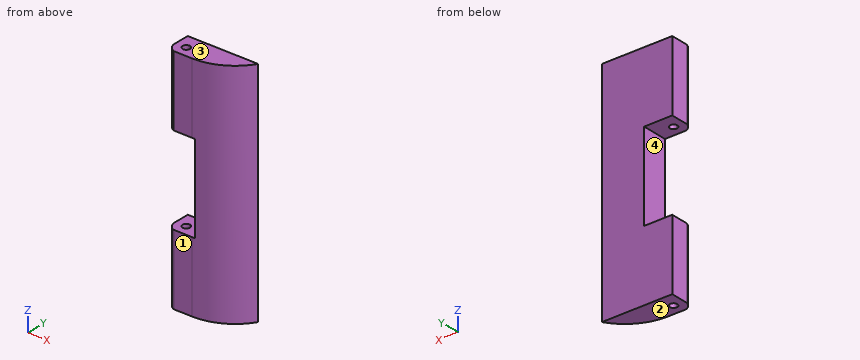
```python
from build123d import *

# Parameters (mm, degrees)
F0_W        = 24
F0_H        = 14.5
F1_DEPTH    = 130
F2_DEPTH    = 130
F3_DEPTH    = 90
F4_DEPTH    = 40
F5_R        = 1
F6_T1_DEPTH = 258.4279953904


# Not quite as in the source:
# - a fillet or chamfer that OpenCascade refuses, or shapes differently, is made with other operations: its cross-section is extruded or revolved along the edge and cut away or added


with BuildPart() as f1:
    # F0 (on Top) → F1 (new body)
    with BuildSketch(Plane.XY):
        with Locations((21.9, 1.16)):
            Rectangle(F0_W, F0_H)
    extrude(amount=F1_DEPTH)

    # F0 (on Top) → F2 (join)
    with BuildSketch(Plane.XY):
        with BuildLine():
            Line((9.9, 8.41), (6.1, 8.41))
            Line((6.1, 8.41), (6.1, -1.59))
            ThreePointArc((6.1, -1.59), (4.7073896383, -4.2954889128), (2.25, -6.09))
            Line((2.25, -6.09), (9.9, -6.09))
            Line((9.9, -6.09), (9.9, 8.41))
        make_face()
        with BuildLine():
            Line((6.1, -1.59), (6.1, 8.41))
            Line((6.1, 8.41), (0, 8.41))
            Line((0, 8.41), (0, 2.15))
            ThreePointArc((0, 2.15), (1.5202795796, 1.5202795796), (2.15, 0))
            ThreePointArc((2.15, 0), (1.5202795796, -1.5202795796), (0, -2.15))
            Line((0, -2.15), (0, -6.09))
            Line((0, -6.09), (2.25, -6.09))
            ThreePointArc((2.25, -6.09), (4.7073896383, -4.2954889128), (6.1, -1.59))
        make_face()
        with BuildLine():
            Line((0, 2.15), (0, 8.41))
            Line((0, 8.41), (-6.1, 8.41))
            Line((-6.1, 8.41), (-6.1, -1.59))
            ThreePointArc((-6.1, -1.59), (-4.7073896383, -4.2954889128), (-2.25, -6.09))
            Line((-2.25, -6.09), (0, -6.09))
            Line((0, -6.09), (0, -2.15))
            ThreePointArc((0, -2.15), (-2.15, 0), (0, 2.15))
        make_face()
    extrude(amount=F2_DEPTH)

    # F0 (on Top) → F3 (cut)
    with BuildSketch(Plane.XY):
        with BuildLine():
            Line((9.9, 8.41), (6.1, 8.41))
            Line((6.1, 8.41), (6.1, -1.59))
            ThreePointArc((6.1, -1.59), (4.7073896383, -4.2954889128), (2.25, -6.09))
            Line((2.25, -6.09), (9.9, -6.09))
            Line((9.9, -6.09), (9.9, 8.41))
        make_face()
        with BuildLine():
            Line((6.1, -1.59), (6.1, 8.41))
            Line((6.1, 8.41), (0, 8.41))
            Line((0, 8.41), (0, 2.15))
            ThreePointArc((0, 2.15), (1.5202795796, 1.5202795796), (2.15, 0))
            ThreePointArc((2.15, 0), (1.5202795796, -1.5202795796), (0, -2.15))
            Line((0, -2.15), (0, -6.09))
            Line((0, -6.09), (2.25, -6.09))
            ThreePointArc((2.25, -6.09), (4.7073896383, -4.2954889128), (6.1, -1.59))
        make_face()
        with BuildLine():
            Line((0, 2.15), (0, 8.41))
            Line((0, 8.41), (-6.1, 8.41))
            Line((-6.1, 8.41), (-6.1, -1.59))
            ThreePointArc((-6.1, -1.59), (-4.7073896383, -4.2954889128), (-2.25, -6.09))
            Line((-2.25, -6.09), (0, -6.09))
            Line((0, -6.09), (0, -2.15))
            ThreePointArc((0, -2.15), (-2.15, 0), (0, 2.15))
        make_face()
    extrude(amount=F3_DEPTH, mode=Mode.SUBTRACT)

    # F0 (on Top) → F4 (join)
    with BuildSketch(Plane.XY):
        with BuildLine():
            Line((0, 2.15), (0, 8.41))
            Line((0, 8.41), (-6.1, 8.41))
            Line((-6.1, 8.41), (-6.1, -1.59))
            ThreePointArc((-6.1, -1.59), (-4.7073896383, -4.2954889128), (-2.25, -6.09))
            Line((-2.25, -6.09), (0, -6.09))
            Line((0, -6.09), (0, -2.15))
            ThreePointArc((0, -2.15), (-2.15, 0), (0, 2.15))
        make_face()
        with BuildLine():
            Line((6.1, -1.59), (6.1, 8.41))
            Line((6.1, 8.41), (0, 8.41))
            Line((0, 8.41), (0, 2.15))
            ThreePointArc((0, 2.15), (1.5202795796, 1.5202795796), (2.15, 0))
            ThreePointArc((2.15, 0), (1.5202795796, -1.5202795796), (0, -2.15))
            Line((0, -2.15), (0, -6.09))
            Line((0, -6.09), (2.25, -6.09))
            ThreePointArc((2.25, -6.09), (4.7073896383, -4.2954889128), (6.1, -1.59))
        make_face()
        with BuildLine():
            Line((9.9, 8.41), (6.1, 8.41))
            Line((6.1, 8.41), (6.1, -1.59))
            ThreePointArc((6.1, -1.59), (4.7073896383, -4.2954889128), (2.25, -6.09))
            Line((2.25, -6.09), (9.9, -6.09))
            Line((9.9, -6.09), (9.9, 8.41))
        make_face()
    extrude(amount=F4_DEPTH)

    # F5
    f5_edges = [f1.edges().sort_by_distance(p)[0] for p in [
        (-2.25, -6.09, 20),
    ]]
    fillet(f5_edges, radius=F5_R)

    # F6: fillet of radius 30 on 1 edges, made by hand

    # F6_s2 → F6_t1 (cut)
    with BuildSketch(Plane.XY.offset(-64.2139976952)):
        with BuildLine():
            ThreePointArc((8.2144009219, -6.09), (22.9622821257, -2.2147009552), (33.9, 8.41))
            Line((33.9, 8.41), (33.9, -6.09))
            Line((33.9, -6.09), (8.2144009219, -6.09))
        make_face()
    extrude(amount=F6_T1_DEPTH, mode=Mode.SUBTRACT)


solid = f1.part
```
Work out the finished part from the listing and answer in its coordinate system (mm). Face numbers are marked on the shaded views. Round coordinates to 2 decimals unless told otherwise and drop trailing zeros. Write each loop counter-clockwise with the first axis right and the second up, starting at its lowest first coordinate (ties: lowest second). Pieces come first, ordered by that corner, then holes. Notation, with made-up numbers: (74.5, 77.5) -> (89.5, 77.5) arc R24 cw to (89.5, 109.5) -> close; hole circle Ø2 at (36, 20.5). An arc over 180 degrees is marked (long way). Write each question's results on one line, items separated by ' | '.
1) The part is cut by section A-A (z = 116). Write down the section's boundary in (x, y).
Findings:
outline: (-6.1, -1.59) arc R6.61 ccw to (-2.25, -6.09) -> (8.21, -6.09) arc R30 ccw to (33.9, 8.41) -> (-6.1, 8.41) -> close; hole circle Ø4.3 at (0, 0)
2) Consider line 1 along Z through (x, y) = (-1.5, 3.75); line 2 along Y through (x, z) = (10.5, 110); line 3 along X through (y, z) = (-1, 30). Determine where each line is inside the solid, lowest interval first. Write a range as [from, to].
Findings:
line 1: z = [0, 40], [90, 130] | line 2: y = [-6, 8.41] | line 3: x = [-6.1, -1.9], [1.9, 24.93]
3) The part is cut by section C-C (x = 24). Write down the section's boundary in (y, z), and give its area (3 significant figures).
Findings:
outline: (-1.6, 0) -> (8.41, 0) -> (8.41, 130) -> (-1.6, 130) -> close | area: 1,300 mm²
4) For a pull along Z with two mould halves and no side action, classify the marked faces 1, 2, 3 and 4 as +Z half, -Z half, draft (parallel to the pull), parting line (faces both ways), or undercut.
Findings:
face 1: draft | face 2: -Z half | face 3: +Z half | face 4: undercut
5) Flat-ended cylindrical pins translate along their axes: pin 1 (7 mm diameter, centred on y = 2.5, z = 65.5, fed in from -X); pin 2 (8 mm diameter, centred on x = 26, z = 63, fed in from -Y) (3 decimals); pin 3 (8 mm diameter, centred on x = 11.5, z = 83.5, fed in from -Y). Find the tip coordinate at first contact, or state that the pin passes through.
Findings:
pin 1: stops at x = 9.9 | pin 2: stops at y = -2.735 | pin 3: stops at y = -6.04
6) The part is cut by section B-B (y = 6.75). Write down the section's boundary in (x, z).
Findings:
outline: (-6.1, 0) -> (32.82, 0) -> (32.82, 130) -> (-6.1, 130) -> (-6.1, 90) -> (9.9, 90) -> (9.9, 40) -> (-6.1, 40) -> close
7) The part is cut by section D-D (z = 66). Write down the section's boundary in (x, y).
Findings:
outline: (9.9, -6.04) arc R30 ccw to (33.9, 8.41) -> (9.9, 8.41) -> close
